from build123d import *

# Parameters (mm, degrees)
SKETCH1_W                 = 85
SKETCH1_H                 = 50
BOSS_EXTRUDE1_DEPTH       = 2.5
SKETCH5_W                 = 22
SKETCH5_H                 = 15
BOSS_EXTRUDE2_DEPTH       = 2.5
LPATTERN4_COUNT           = 2
LPATTERN4_PITCH           = 63
LPATTERN5_COUNT           = 2
LPATTERN5_PITCH           = 65
LPATTERN5_COPY_1_SKETCH_W = 22
LPATTERN5_COPY_1_SKETCH_H = 15
LPATTERN5_COPY_1_DEPTH    = 2.5
SKETCH2_W                 = 3
SKETCH2_H                 = 70
CUT_EXTRUDE1_DEPTH        = 2.5
LPATTERN1_COUNT           = 2
LPATTERN1_PITCH           = 62
SKETCH3_R                 = 11.25
CUT_EXTRUDE2_DEPTH        = 108.033873143
SKETCH4_R                 = 1.5
CUT_EXTRUDE3_DEPTH        = 108.033873143
LPATTERN2_COUNT           = 2
LPATTERN2_PITCH           = 31
LPATTERN3_COUNT           = 2
LPATTERN3_PITCH           = 31
LPATTERN3_COPY_1_SKETCH_R = 1.5
LPATTERN3_COPY_1_DEPTH    = 108.033873143


with BuildPart() as part:
    # Sketch1 → Boss-Extrude1 (new body)
    with BuildSketch(Plane.XY):
        with Locations((42.5, 25)):
            Rectangle(SKETCH1_W, SKETCH1_H)
    extrude(amount=BOSS_EXTRUDE1_DEPTH)

    # Sketch5 → Boss-Extrude2 (add)
    with BuildSketch(Plane.XY):
        with Locations((11, 57.5)):
            Rectangle(SKETCH5_W, SKETCH5_H)
    boss_extrude2 = extrude(amount=BOSS_EXTRUDE2_DEPTH)

    # LPattern4: Boss-Extrude2 ×2
    with Locations(*[(i * LPATTERN4_PITCH, 0, 0) for i in range(1, LPATTERN4_COUNT)]):
        add(boss_extrude2)

    # LPattern5: Boss-Extrude2 ×2
    with Locations(*[(0, -i * LPATTERN5_PITCH, 0) for i in range(1, LPATTERN5_COUNT)]):
        add(boss_extrude2)

    # LPattern5 copy 1 sketch → LPattern5 copy 1 (add)
    with BuildSketch(Plane(origin=(63, -65, 0), x_dir=(1, 0, 0), z_dir=(0, 0, 1))):
        with Locations((11, 57.5)):
            Rectangle(LPATTERN5_COPY_1_SKETCH_W, LPATTERN5_COPY_1_SKETCH_H)
    extrude(amount=LPATTERN5_COPY_1_DEPTH)

    # Sketch2 → Cut-Extrude1 (cut)
    with BuildSketch(Plane.XY.offset(2.5)):
        with Locations((6.5, 25)):
            Rectangle(SKETCH2_W, SKETCH2_H)
        with Locations((16.5, 25)):
            Rectangle(SKETCH2_W, SKETCH2_H)
    cut_extrude1 = extrude(amount=-CUT_EXTRUDE1_DEPTH, mode=Mode.SUBTRACT)

    # LPattern1: Cut-Extrude1 ×2
    with Locations(*[(i * LPATTERN1_PITCH, 0, 0) for i in range(1, LPATTERN1_COUNT)]):
        add(cut_extrude1, mode=Mode.SUBTRACT)

    # Sketch3 → Cut-Extrude2 (cut, through all)
    with BuildSketch(Plane.XY.offset(2.5)):
        with Locations((42.5, 25)):
            Circle(SKETCH3_R)
    extrude(amount=-CUT_EXTRUDE2_DEPTH, mode=Mode.SUBTRACT)

    # Sketch4 → Cut-Extrude3 (cut, through all)
    with BuildSketch(Plane.XY.offset(2.5)):
        with Locations((27, 40.5)):
            Circle(SKETCH4_R)
    cut_extrude3 = extrude(amount=-CUT_EXTRUDE3_DEPTH, mode=Mode.SUBTRACT)

    # LPattern2: Cut-Extrude3 ×2
    with Locations(*[(0, -i * LPATTERN2_PITCH, 0) for i in range(1, LPATTERN2_COUNT)]):
        add(cut_extrude3, mode=Mode.SUBTRACT)

    # LPattern3: Cut-Extrude3 ×2
    with Locations(*[(i * LPATTERN3_PITCH, 0, 0) for i in range(1, LPATTERN3_COUNT)]):
        add(cut_extrude3, mode=Mode.SUBTRACT)

    # LPattern3 copy 1 sketch → LPattern3 copy 1 (cut, through all)
    with BuildSketch(Plane(origin=(31, -31, 2.5), x_dir=(1, 0, 0), z_dir=(0, 0, 1))):
        with Locations((27, 40.5)):
            Circle(LPATTERN3_COPY_1_SKETCH_R)
    extrude(amount=-LPATTERN3_COPY_1_DEPTH, mode=Mode.SUBTRACT)


solid = part.part
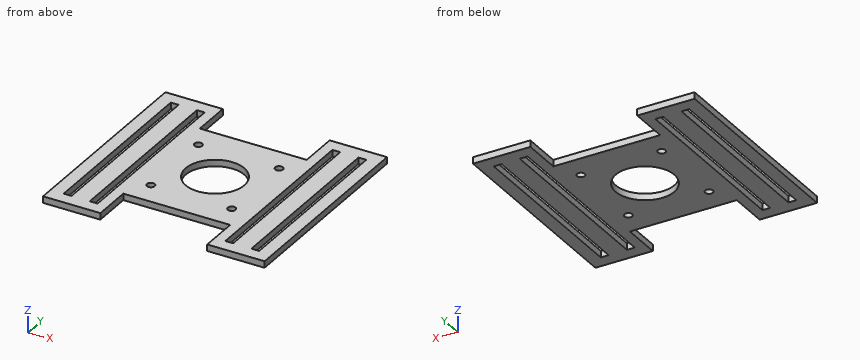
Can you work these out from the model? Positions are in its coordinate system, mm. Give positions to 0.01 mm unless a question says otherwise; leave off trailing zeros. Order: outer loops, then holes, each group sorted by start corner. A loop starts at its lowest first (then second) coordinate and runs counter-clockwise, first axis right, second up. Notation, with made-up numbers: M 80.5,37 L 121.5,37 A6 ccw 121.5,44 Z; hole C 62,-6.5 d11. An arc over 180 degrees is marked long. Use one line per item in the form item = value. Start each with the question number.
Item 1: If I drill on line 1 along Y through (x, z) = (27, 1.55); line 2 along X through (y, z) = (5.5, 1); line 3 along X through (y, z) = (58, 1.9), over which ranges is the centre line in solid material (lowest first)?
Item 2: If we section it at C-C (x = 16): Write out the boundary of the cut face in (y, z), then the cut area to 3 significant figures.
Item 3: If we section it at B-B (x = 27): Write out the boundary of the cut face in (y, z).
Item 4: If we section it at D-D (z = 2): State how many separate pieces and enclosed holes the cut face has, then the cut area to 3 significant figures.
Item 5: Will this pin go through, and if not, where does the flat tip stop? pin 1 Ø1 at (x, z) = (26.5, 0.5) entering from -Y.
Item 6: If we section it at A-A (y = -3): Write out the boundary of the cut face in (x, z), then the cut area to 3 significant figures.
Outcome:
q1.line_1 = 0 to 8, 11 to 39, 42 to 50
q1.line_2 = 0 to 5, 8 to 15, 18 to 67, 70 to 77, 80 to 85
q1.line_3 = 0 to 5, 8 to 15, 18 to 22, 63 to 67, 70 to 77, 80 to 85
q2.outline = M -15,0 L -10,0 L -10,2.5 L -15,2.5 Z; M 60,0 L 65,0 L 65,2.5 L 60,2.5 Z
q2.area = 25.0 mm2
q3.outline = M 0,0 L 8,0 L 8,2.5 L 0,2.5 Z; M 11,0 L 39,0 L 39,2.5 L 11,2.5 Z; M 42,0 L 50,0 L 50,2.5 L 42,2.5 Z
q4.separate_pieces = 1
q4.enclosed_holes = 9
q4.area = 4,300 mm2
q5.pin_1 = 0
q6.outline = M 0,0 L 5,0 L 5,2.5 L 0,2.5 Z; M 8,0 L 15,0 L 15,2.5 L 8,2.5 Z; M 18,0 L 22,0 L 22,2.5 L 18,2.5 Z; M 63,0 L 67,0 L 67,2.5 L 63,2.5 Z; M 70,0 L 77,0 L 77,2.5 L 70,2.5 Z; M 80,0 L 85,0 L 85,2.5 L 80,2.5 Z
q6.area = 80.0 mm2
